Verification items for the finished model (mm, model axes). Face numbers are marked on the shaded views. Give positions to 0.01 mm unless a question says otherwise; leave off trailing zeros. Write each loop counter-clockwise with the first axis right and the second up, starting at its lowest first coordinate (ties: lowest second). Pieces come first, ordered by that corner, then holes. Notation, with made-up numbers: (-14, 71.25) -> (31, 71.25) arc R20 cw to (31, 75.25) -> close; hole circle Ø2 at (86.25, 78). An arc over 180 degrees is marked (long way). Use one line per item in the form item = value. Start each with the question number.
(1) Scan lines: L1, parallel to X at y = -46, z = 29.5; L2, parallel to Z at x = -433.5, y = -4.5; L3, parallel to Y at x = 539.5, z = 6. Record each from-to range of solid material in increasing order.
(2) Release check for a two-part mould opening along Z. For the marked faces 1 and 2 record: pulls with the +Z half, pulls with the -Z half, needs draft (parallel to the pull), parting line crosses it, or undercut.
(3) Depth check by flat-ended pin: pin 1 Ø5 at (x, y) = (-615, -77.5) entering from +Z; pin 2 Ø14.5 at (y, z) = (-5.5, 5) entering from +X; pin 3 Ø4 at (x, z) = (142.5, 44.5) entering from -Y. Enter the tip coordinate at first touch or a pass-through.
(4) Section check C-C, the plane x = 21.5. Record the cut outline in (y, z), plus the area to 3 significant figures.
(5) Section check A-A, the plane y = -61. Record the cut outline in (x, z).
(6) Section check B-B, the plane z = 59.5. Record the cut outline in (x, y).
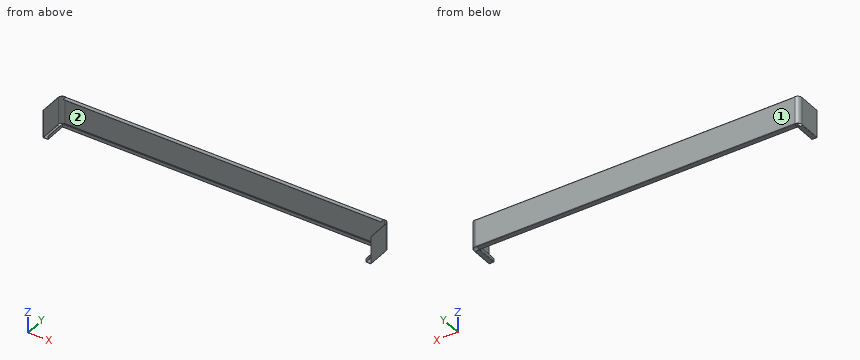
from build123d import *

# Parameters (mm, degrees)
BASE_FLANGE1_DEPTH            = 104
EDGE_FLANGE1_STRIP_W          = 6
EDGE_FLANGE1_STRIP_H          = 1
EDGE_FLANGE1_STRIP_CUT_DEPTH  = 1204
EDGE_FLANGE1_RELIEF_W         = 6.5
EDGE_FLANGE1_RELIEF_H         = 0.5
EDGE_FLANGE1_RELIEF_CUT_DEPTH = 1
EDGE_FLANGE1_DEPTH            = 1204
EDGE_FLANGE2_STRIP_W          = 6
EDGE_FLANGE2_STRIP_H          = 1
EDGE_FLANGE2_STRIP_CUT_DEPTH  = 1204
EDGE_FLANGE2_DEPTH            = 1204
EDGE_FLANGE3_STRIP_W          = 6
EDGE_FLANGE3_STRIP_H          = 1
EDGE_FLANGE3_STRIP_CUT_DEPTH  = 80
EDGE_FLANGE3_RELIEF_W         = 6.5
EDGE_FLANGE3_RELIEF_H         = 0.5
EDGE_FLANGE3_RELIEF_CUT_DEPTH = 1
EDGE_FLANGE3_DEPTH            = 80
EDGE_FLANGE4_STRIP_W          = 6
EDGE_FLANGE4_STRIP_H          = 1
EDGE_FLANGE4_STRIP_CUT_DEPTH  = 80
EDGE_FLANGE4_DEPTH            = 80
EDGE_FLANGE5_STRIP_W          = 6
EDGE_FLANGE5_STRIP_H          = 1
EDGE_FLANGE5_STRIP_CUT_DEPTH  = 1204
EDGE_FLANGE5_RELIEF_W         = 6.5
EDGE_FLANGE5_RELIEF_H         = 0.5
EDGE_FLANGE5_RELIEF_CUT_DEPTH = 1
EDGE_FLANGE5_DEPTH            = 1204


# Sheet-metal steps are written as plain solids
with BuildPart() as part:
    # Sketch1 → Base-Flange1 (new body)
    with BuildSketch(Plane.XY):
        with BuildLine():
            Line((-621, -100), (-621, -15))
            ThreePointArc((-621, -15), (-616.606601718, -4.393398282), (-606, 0))
            Line((-606, 0), (606, 0))
            ThreePointArc((606, 0), (616.606601718, -4.393398282), (621, -15))
            Line((621, -15), (621, -100))
            Line((621, -100), (622, -100))
            Line((622, -100), (622, -15))
            ThreePointArc((622, -15), (617.313708499, -3.686291501), (606, 1))
            Line((606, 1), (-606, 1))
            ThreePointArc((-606, 1), (-617.313708499, -3.686291501), (-622, -15))
            Line((-622, -15), (-622, -100))
            Line((-622, -100), (-621, -100))
        make_face()
    extrude(amount=BASE_FLANGE1_DEPTH)

    # Edge-Flange1 strip (across the edge) → Edge-Flange1 strip cut (cut)
    with BuildSketch(Plane(origin=(-602, 0, 0), x_dir=(0, 0, 1), z_dir=(1, 0, 0))):
        with Locations((-2, -0.5)):
            Rectangle(EDGE_FLANGE1_STRIP_W, EDGE_FLANGE1_STRIP_H)
    extrude(amount=EDGE_FLANGE1_STRIP_CUT_DEPTH, mode=Mode.SUBTRACT)

    # Edge-Flange1 relief (on the sheet) → Edge-Flange1 relief cut (cut)
    with BuildSketch(Plane(origin=(-602, 0, 1), x_dir=(0, 0, 1), z_dir=(0, -1, 0))):
        with Locations((-2.75, 0.25)):
            Rectangle(EDGE_FLANGE1_RELIEF_W, EDGE_FLANGE1_RELIEF_H)
        with Locations((-2.75, -1204.25)):
            Rectangle(EDGE_FLANGE1_RELIEF_W, EDGE_FLANGE1_RELIEF_H)
    extrude(amount=-EDGE_FLANGE1_RELIEF_CUT_DEPTH, mode=Mode.SUBTRACT)

    # Edge-Flange1 section (across the edge) → Edge-Flange1 (add)
    with BuildSketch(Plane(origin=(-602, 0, 0), x_dir=(0, 0, 1), z_dir=(1, 0, 0))):
        with BuildLine():
            Line((-1, 1), (-1, 19))
            Line((-1, 19), (0, 19))
            Line((0, 19), (0, 1))
            ThreePointArc((0, 1), (0.292893219, 0.292893219), (1, 0))
            Line((1, 0), (1, -1))
            ThreePointArc((1, -1), (-0.414213562, -0.414213562), (-1, 1))
        make_face()
    extrude(amount=EDGE_FLANGE1_DEPTH)

    # Edge-Flange2 strip (across the edge) → Edge-Flange2 strip cut (cut)
    with BuildSketch(Plane(origin=(-602, -19, 0), x_dir=(0, 1, 0), z_dir=(1, 0, 0))):
        with Locations((-1, -0.5)):
            Rectangle(EDGE_FLANGE2_STRIP_W, EDGE_FLANGE2_STRIP_H)
    extrude(amount=EDGE_FLANGE2_STRIP_CUT_DEPTH, mode=Mode.SUBTRACT)

    # Edge-Flange2 section (across the edge) → Edge-Flange2 (add)
    with BuildSketch(Plane(origin=(-602, -19, 0), x_dir=(0, 1, 0), z_dir=(1, 0, 0))):
        with BuildLine():
            Line((0, 1), (0, 12))
            Line((0, 12), (1, 12))
            Line((1, 12), (1, 1))
            ThreePointArc((1, 1), (1.292893219, 0.292893219), (2, 0))
            Line((2, 0), (2, -1))
            ThreePointArc((2, -1), (0.585786438, -0.414213562), (0, 1))
        make_face()
    extrude(amount=EDGE_FLANGE2_DEPTH)

    # Edge-Flange3 strip (across the edge) → Edge-Flange3 strip cut (cut)
    with BuildSketch(Plane(origin=(-621, -100, 0), x_dir=(0, 0, 1), z_dir=(0, 1, 0))):
        with Locations((-2, -0.5)):
            Rectangle(EDGE_FLANGE3_STRIP_W, EDGE_FLANGE3_STRIP_H)
    edge_flange3_strip_cut = extrude(amount=EDGE_FLANGE3_STRIP_CUT_DEPTH, mode=Mode.SUBTRACT)

    # Edge-Flange3 relief (on the sheet) → Edge-Flange3 relief cut (cut)
    with BuildSketch(Plane(origin=(-621, -100, 1), x_dir=(0, 0, 1), z_dir=(1, 0, 0))):
        with Locations((-2.75, -80.25)):
            Rectangle(EDGE_FLANGE3_RELIEF_W, EDGE_FLANGE3_RELIEF_H)
    edge_flange3_relief_cut = extrude(amount=-EDGE_FLANGE3_RELIEF_CUT_DEPTH, mode=Mode.SUBTRACT)

    # Edge-Flange3 section (across the edge) → Edge-Flange3 (add)
    with BuildSketch(Plane(origin=(-621, -100, 0), x_dir=(0, 0, 1), z_dir=(0, 1, 0))):
        with BuildLine():
            Line((-1, 1), (-1, 19))
            Line((-1, 19), (0, 19))
            Line((0, 19), (0, 1))
            ThreePointArc((0, 1), (0.292893219, 0.292893219), (1, 0))
            Line((1, 0), (1, -1))
            ThreePointArc((1, -1), (-0.414213562, -0.414213562), (-1, 1))
        make_face()
    edge_flange3 = extrude(amount=EDGE_FLANGE3_DEPTH)

    # Edge-Flange4 strip (across the edge) → Edge-Flange4 strip cut (cut)
    with BuildSketch(Plane(origin=(-602, -100, 0), x_dir=(-1, 0, 0), z_dir=(0, 1, 0))):
        with Locations((-1, -0.5)):
            Rectangle(EDGE_FLANGE4_STRIP_W, EDGE_FLANGE4_STRIP_H)
    edge_flange4_strip_cut = extrude(amount=EDGE_FLANGE4_STRIP_CUT_DEPTH, mode=Mode.SUBTRACT)

    # Edge-Flange4 section (across the edge) → Edge-Flange4 (add)
    with BuildSketch(Plane(origin=(-602, -100, 0), x_dir=(-1, 0, 0), z_dir=(0, 1, 0))):
        with BuildLine():
            Line((0, 1), (0, 12))
            Line((0, 12), (1, 12))
            Line((1, 12), (1, 1))
            ThreePointArc((1, 1), (1.292893219, 0.292893219), (2, 0))
            Line((2, 0), (2, -1))
            ThreePointArc((2, -1), (0.585786438, -0.414213562), (0, 1))
        make_face()
    edge_flange4 = extrude(amount=EDGE_FLANGE4_DEPTH)

    # Mirror1: Edge-Flange3 strip cut, Edge-Flange3 relief cut, Edge-Flange3, Edge-Flange4 strip cut, Edge-Flange4 across plane
    add(edge_flange3_strip_cut.mirror(Plane(origin=(0, 0, 0), x_dir=(0, 0, 1), z_dir=(1, 0, 0))), mode=Mode.SUBTRACT)
    add(edge_flange3_relief_cut.mirror(Plane(origin=(0, 0, 0), x_dir=(0, 0, 1), z_dir=(1, 0, 0))), mode=Mode.SUBTRACT)
    add(edge_flange3.mirror(Plane(origin=(0, 0, 0), x_dir=(0, 0, 1), z_dir=(1, 0, 0))))
    add(edge_flange4_strip_cut.mirror(Plane(origin=(0, 0, 0), x_dir=(0, 0, 1), z_dir=(1, 0, 0))), mode=Mode.SUBTRACT)
    add(edge_flange4.mirror(Plane(origin=(0, 0, 0), x_dir=(0, 0, 1), z_dir=(1, 0, 0))))

    # Edge-Flange5 strip (across the edge) → Edge-Flange5 strip cut (cut)
    with BuildSketch(Plane(origin=(602, 0, 104), x_dir=(0, 0, -1), z_dir=(-1, 0, 0))):
        with Locations((-1, -0.5)):
            Rectangle(EDGE_FLANGE5_STRIP_W, EDGE_FLANGE5_STRIP_H)
    extrude(amount=EDGE_FLANGE5_STRIP_CUT_DEPTH, mode=Mode.SUBTRACT)

    # Edge-Flange5 relief (on the sheet) → Edge-Flange5 relief cut (cut)
    with BuildSketch(Plane(origin=(602, 0, 102), x_dir=(0, 0, -1), z_dir=(0, -1, 0))):
        with Locations((-2.75, 0.25)):
            Rectangle(EDGE_FLANGE5_RELIEF_W, EDGE_FLANGE5_RELIEF_H)
        with Locations((-2.75, -1204.25)):
            Rectangle(EDGE_FLANGE5_RELIEF_W, EDGE_FLANGE5_RELIEF_H)
    extrude(amount=-EDGE_FLANGE5_RELIEF_CUT_DEPTH, mode=Mode.SUBTRACT)

    # Edge-Flange5 section (across the edge) → Edge-Flange5 (add)
    with BuildSketch(Plane(origin=(602, 0, 104), x_dir=(0, 0, -1), z_dir=(-1, 0, 0))):
        with BuildLine():
            Line((0, 1), (0, 15))
            Line((0, 15), (1, 15))
            Line((1, 15), (1, 1))
            ThreePointArc((1, 1), (1.292893219, 0.292893219), (2, 0))
            Line((2, 0), (2, -1))
            ThreePointArc((2, -1), (0.585786438, -0.414213562), (0, 1))
        make_face()
    extrude(amount=EDGE_FLANGE5_DEPTH)


solid = part.part
Completed:
q1.L1 = -622 to -621, 621 to 622
q1.L2 = -1 to 0, 103 to 104
q1.L3 = -19 to -18, 0 to 1
q2.face_1 = needs draft
q2.face_2 = undercut
q3.pin_1 = 0
q3.pin_2 = 621.84
q3.pin_3 = 0
q4.outline = (-19, 1) arc R2 ccw to (-17, -1) -> (-1, -1) arc R2 ccw to (1, 1) -> (1, 102) arc R2 ccw to (-1, 104) -> (-15, 104) -> (-15, 103) -> (-1, 103) arc R1 cw to (0, 102) -> (0, 1) arc R1 cw to (-1, 0) -> (-17, 0) arc R1 cw to (-18, 1) -> (-18, 12) -> (-19, 12) -> close
q4.area = 149 mm²
q5.outline = (-622, 1) arc R2 ccw to (-620, -1) -> (-604, -1) arc R2 ccw to (-602, 1) -> (-602, 12) -> (-603, 12) -> (-603, 1) arc R1 cw to (-604, 0) -> (-620, 0) arc R1 cw to (-621, 1) -> (-621, 104) -> (-622, 104) -> close; (602, 1) arc R2 ccw to (604, -1) -> (620, -1) arc R2 ccw to (622, 1) -> (622, 104) -> (621, 104) -> (621, 1) arc R1 cw to (620, 0) -> (604, 0) arc R1 cw to (603, 1) -> (603, 12) -> (602, 12) -> close
q6.outline = (-622, -100) -> (-621, -100) -> (-621, -15) arc R15 cw to (-606, 0) -> (606, 0) arc R15 cw to (621, -15) -> (621, -100) -> (622, -100) -> (622, -15) arc R16 ccw to (606, 1) -> (-606, 1) arc R16 ccw to (-622, -15) -> close
